Can you work these out from the model? Positions are in its coordinate system, mm. A direction names the side the tool comes from. Give positions to 0.01 mm unless a question says otherwise; leave off trailing zeros. Order: outer loops, then holes, each group sorted by start corner. A loop starts at its lowest first (then second) coordinate and runs counter-clockwise, first axis right, second up. Notation, with made-up numbers: (-12.75, -27.5) -> (5.25, -27.5) arc R14 ccw to (5.25, -4.5) -> close; hole circle Ø2 at (-33, 34). An arc over 180 degrees is marked (long way). Answer as CSV lines item,"result".
Autodesk Inventor part; units mm, degrees
ref_plane "YZ Plane" through (0, 0, 0) normal (1, 0, 0) x (0, 1, 0)
ref_plane "XZ Plane" through (0, 0, 0) normal (0, 1, 0) x (-1, 0, 0)
ref_plane "XY Plane" through (0, 0, 0) normal (0, 0, 1) x (1, 0, 0)
sketch "Sketch1" plane through (0, 0, 0) normal (0, 0, 1) x (1, 0, 0)
  line L0 (-12.5, -10) -> (12.5, -10)
  line L1 (12.5, -10) -> (12.5, 10)
  line L2 (12.5, 10) -> (-12.5, 10)
  line L3 (-12.5, 10) -> (-12.5, -10)
  line L4 (-12.5, -10) -> (12.5, 10) construction
  line L5 (12.5, -10) -> (-12.5, 10) construction
  line L6 (-12.5, 10) -> (-10, 10)
  line L7 (-10, 10) -> (-10, -10)
  line L8 (-10, -10) -> (-12.5, -10)
  line L9 (-12.5, -10) -> (-12.5, 10)
  line L10 (12.5, -10) -> (10, -10)
  line L11 (10, -10) -> (10, 10)
  line L12 (10, 10) -> (12.5, 10)
  line L13 (12.5, 10) -> (12.5, -10)
  point P0 (0, 0)
  point P1 (0, 0)
  dimension "d0" = 25
  dimension "d1" = 20
  dimension "d2" = 2.5
  dimension "d3" = 2.5
extrude "Extrusion1" add sketch "Sketch1" along normal blind 2.5 contours L7 L2 L11 L0
extrude "Extrusion2" add sketch "Sketch1" along normal blind 30.5 contours L3 L2 L7 L0 | L11 L2 L1 L0
hole "Hole1" at (0, 0, 0) direction (0, 0, 1) diameter 4.5 end through all both
properties part number "slotcar_beam"
Item 1: Imagine slicing it at A-A, the plane y = 0. Please give me the cut outline in (x, z).
Numbers:
outline,"(-12.5, 0) -> (-2.25, 0) -> (-2.25, 2.5) -> (-10, 2.5) -> (-10, 30.5) -> (-12.5, 30.5) -> close; (2.25, 0) -> (12.5, 0) -> (12.5, 30.5) -> (10, 30.5) -> (10, 2.5) -> (2.25, 2.5) -> close"
Item 2: We'd pull the mould along X, two halves only. Please class faces 1 (the flat face through (-10.2, -10, 11.8)), 2 (the flat face through (-10, 0, 16)), 3 (the flat face through (12.5, 0, 15)): released by +X, released by -X, zero draft, split by the parting line, or undercut.
Numbers:
face 1,"zero draft"
face 2,"undercut"
face 3,"released by +X"
Item 3: Imagine slicing it at B-B, the plane x = 0. Please give me the cut outline in (y, z).
Numbers:
outline,"(-10, 0) -> (-2.25, 0) -> (-2.25, 2.5) -> (-10, 2.5) -> close; (2.25, 0) -> (10, 0) -> (10, 2.5) -> (2.25, 2.5) -> close"
Item 4: For pin 1 (12 mm diameter, centred on x = 3, y = -6.5, fed in from +Z); pin 2 (10 mm diameter, centred on x = 9.5, z = 10, fed in from +Y), each with a flat end and sliding along its axis, tell me the tip position at first contact or that it passes through.
Numbers:
pin 1,"stops at z = 2.5"
pin 2,"stops at y = 10"
Item 5: Please list where these lines run through material, in increasing order: line 1 along X through (y, z) = (3.25, 6.5); line 2 along Y through (x, z) = (0, 1.7); line 3 along X through (y, z) = (0, 1.05).
Numbers:
line 1,"x = -12.5 to -10, 10 to 12.5"
line 2,"y = -10 to -2.25, 2.25 to 10"
line 3,"x = -12.5 to -2.25, 2.25 to 12.5"
Item 6: For faces 4 (the flat face through (-11, 0, 30.5)), 5 (the flat face through (10, 0, 16)), which set-ups out of +Z, -Z, +X, -X, +Y, -Y let a thin tool reach every point of the face, with its end or its side?
Numbers:
face 4,"+Z, +X, -X, +Y, -Y"
face 5,"+Z, +Y, -Y"
Item 7: Imagine slicing it at C-C, the plane z = 9.5. Please give me the cut outline in (x, y), then the cut area to 3 significant figures.
Numbers:
outline,"(-12.5, -10) -> (-10, -10) -> (-10, 10) -> (-12.5, 10) -> close; (10, -10) -> (12.5, -10) -> (12.5, 10) -> (10, 10) -> close"
area,"100 mm²"
Item 8: Imagine slicing it at D-D, the plane y = -3. Please give me the cut outline in (x, z), then the cut area to 4 significant figures.
Numbers:
outline,"(-12.5, 0) -> (12.5, 0) -> (12.5, 30.5) -> (10, 30.5) -> (10, 2.5) -> (-10, 2.5) -> (-10, 30.5) -> (-12.5, 30.5) -> close"
area,"202.5 mm²"
